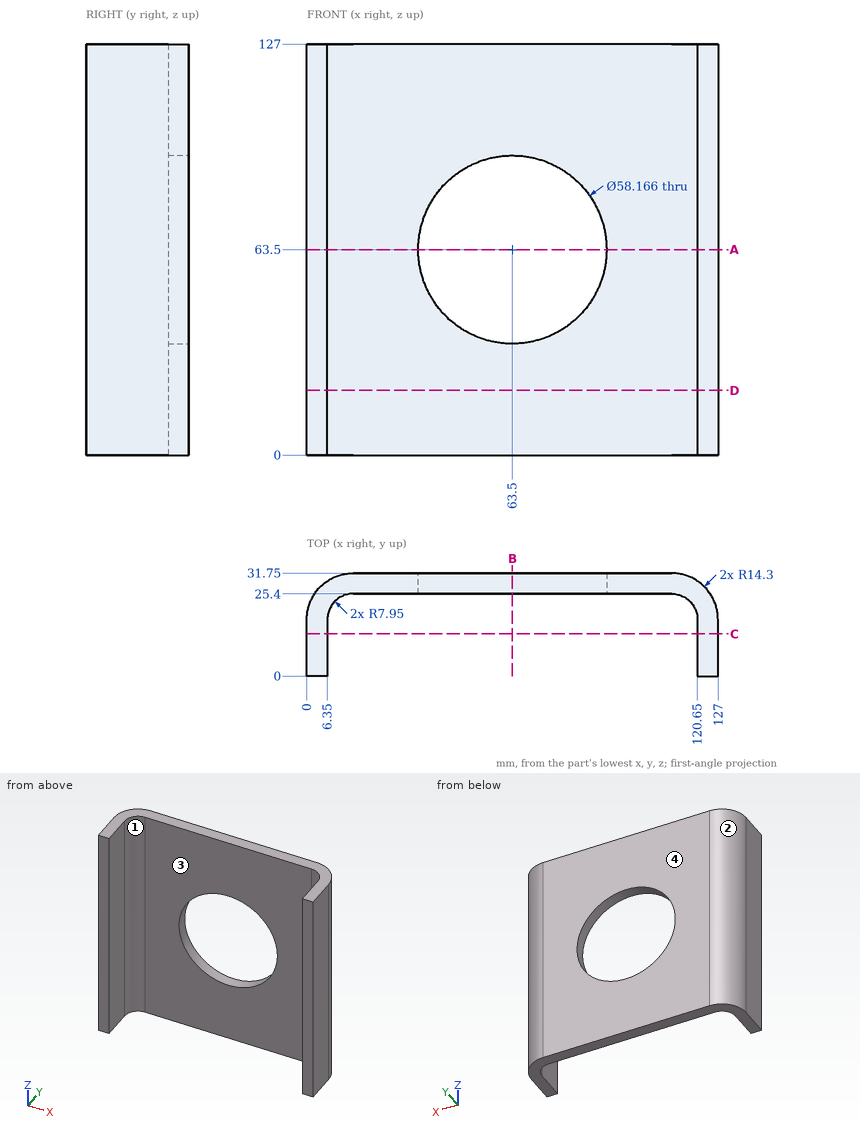
The figure shows three views and two pictorial views of one solid part (mm, origin at its lowest corner). Answer the questions. Coordinates: 2 decimals unless noted, no trailing zeros. Loops run counter-clockwise (first coordinate to the right, second up) from the corner with the lowest first, then second, coordinate; pieces in that order, holes last. Notation, with made-up numbers: (48, 75.5) - (84, 75.5) arc R24 ccw to (84, 108.5) - close; hole circle Ø5 at (84.5, 14.5). An arc over 180 degrees is marked (long way). Answer in a Markdown table with one row per item.
Q1. Find section C-C on y = 13. Write down the section's boundary in (x, z), plus the area to 3 significant figures.
Here are the results:
| item | result |
|---|---|
| outline | (0, 0) - (6.35, 0) - (6.35, 127) - (0, 127) - close; (120.65, 0) - (127, 0) - (127, 127) - (120.65, 127) - close |
| area | 1,610 mm^2 |
Q2. Find section B-B on x = 63.5. Write down the section's boundary in (y, z), plus the area to 3 significant figures.
Here are the results:
| item | result |
|---|---|
| outline | (25.4, 0) - (31.75, 0) - (31.75, 34.42) - (25.4, 34.42) - close; (25.4, 92.58) - (31.75, 92.58) - (31.75, 127) - (25.4, 127) - close |
| area | 437 mm^2 |
Q3. Find section D-D on z = 20. Write down the section's boundary in (x, y), plus the area to 3 significant figures.
Here are the results:
| item | result |
|---|---|
| outline | (0, 0) - (6.35, 0) - (6.35, 17.45) arc R7.95 cw to (14.3, 25.4) - (112.7, 25.4) arc R7.95 cw to (120.65, 17.45) - (120.65, 0) - (127, 0) - (127, 17.45) arc R14.3 ccw to (112.7, 31.75) - (14.3, 31.75) arc R14.3 ccw to (0, 17.45) - close |
| area | 1,070 mm^2 |
Q4. Find section A-A on z = 63.5. Write down the section's boundary in (x, y).
Here are the results:
| item | result |
|---|---|
| outline | (0, 0) - (6.35, 0) - (6.35, 17.45) arc R7.95 cw to (14.3, 25.4) - (34.42, 25.4) - (34.42, 31.75) - (14.3, 31.75) arc R14.3 ccw to (0, 17.45) - close; (92.58, 25.4) - (112.7, 25.4) arc R7.95 cw to (120.65, 17.45) - (120.65, 0) - (127, 0) - (127, 17.45) arc R14.3 ccw to (112.7, 31.75) - (92.58, 31.75) - close |
Q5. Straight lines are drawn through the part: line 1 along Z through (x, y) = (63.5, 29.5); line 2 along X through (y, z) = (13.5, 101.5); line 3 along Y through (x, z) = (108.5, 6). For each, find the intervals that lie inside material, in ascending order. Write a range as [from, to].
Here are the results:
| item | result |
|---|---|
| line 1 | z = [0, 34.42], [92.58, 127] |
| line 2 | x = [0, 6.35], [120.65, 127] |
| line 3 | y = [25.4, 31.75] |
Q6. Given P1, Ø1, axis at x = 89.5, z = 106, coming from the -Y side; P2, Ø12, axis at x = 109, z = 64.5, coming from the -Y side; P3, Ø5, axis at x = 69.5, y = 24.5, coming from the +Z side; P4, Ø2, axis at y = 22, z = 20.5, coming from the -X side, each flat-ended and moving along its own axis, determine where each tip first touches the part or whether it passes through.
Here are the results:
| item | result |
|---|---|
| P1 | stops at y = 25.4 |
| P2 | stops at y = 25.06 |
| P3 | stops at z = 127 |
| P4 | stops at x = 0.45 |
Q7. The mould has two halves that part along X. Classify the marked faces 1, 2, 3 and 4: pulls with the +X half, pulls with the -X half, needs draft (parallel to the pull), parting line crosses it, or undercut.
Here are the results:
| item | result |
|---|---|
| face 1 | undercut |
| face 2 | pulls with the -X half |
| face 3 | undercut |
| face 4 | needs draft |
